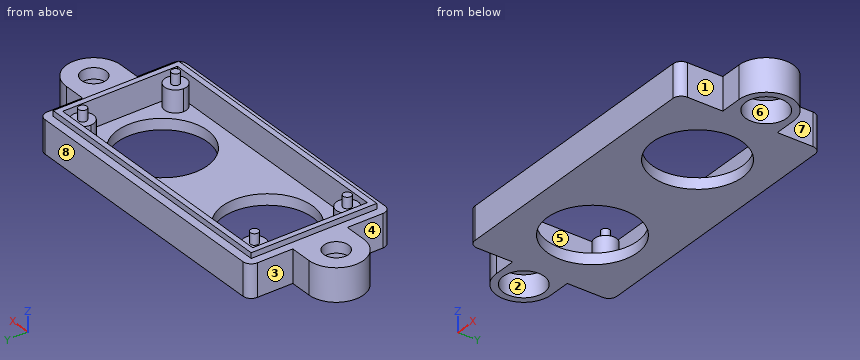
from build123d import *

# Parameters (mm, degrees)
SKETCH011_R             = 2.25
PAD004_DEPTH            = 6
SKETCH021_W             = 49
SKETCH021_H             = 23
SKETCH021_W_2           = 47
SKETCH021_H_2           = 21
PAD005_DEPTH            = 1
SKETCH020_W             = 47
SKETCH020_H             = 21
POCKET005_DEPTH         = 4
SKETCH012_R             = 8.25
POCKET006_DEPTH         = 8
POCKET006_DEPTH_BACK    = 8
SKETCH022_R             = 3.75
POCKET007_DEPTH         = 4
SKETCH024_R             = 2
PAD006_DEPTH            = 6
SKETCH025_R             = 0.75
PAD007_DEPTH            = 2
FILLET001_R             = 1.5
BODY001_PLACEMENT_ANGLE = 180


with BuildPart() as part:
    # Sketch011 → Pad004 (new body)
    with BuildSketch(Plane.XY):
        with BuildLine():
            Line((-26, 13), (26, 13))
            Line((26, 13), (26, 5))
            Line((30, 5), (26, 5))
            ThreePointArc((29.999982, -5), (35, -9e-06), (30, 5))
            Line((29.999982, -5), (25.999982, -5))
            Line((25.999982, -5), (25.999982, -13))
            Line((-26, -13), (25.999982, -13))
            Line((-26, -5), (-26, -13))
            Line((-30, -5), (-26, -5))
            ThreePointArc((-30, 5), (-35, 0), (-30, -5))
            Line((-30, 5), (-26, 5))
            Line((-26, 13), (-26, 5))
        make_face()
        with Locations((-30, 0)):
            Circle(SKETCH011_R, mode=Mode.SUBTRACT)
        with Locations((30, 0)):
            Circle(SKETCH011_R, mode=Mode.SUBTRACT)
    extrude(amount=PAD004_DEPTH)

    # Sketch021 → Pad005 (join, symmetric)
    with BuildSketch(Plane.XY):
        Rectangle(SKETCH021_W, SKETCH021_H)
        Rectangle(SKETCH021_W_2, SKETCH021_H_2, mode=Mode.SUBTRACT)
    extrude(amount=PAD005_DEPTH, both=True)

    # Sketch020 → Pocket005 (cut)
    with BuildSketch(Plane.XY):
        Rectangle(SKETCH020_W, SKETCH020_H)
    extrude(amount=POCKET005_DEPTH, mode=Mode.SUBTRACT)

    # Sketch012 → Pocket006 (cut, two sides)
    with BuildSketch(Plane.XY) as pocket006_sk:
        with Locations((-13, 0)):
            Circle(SKETCH012_R)
        with Locations((13, 0)):
            Circle(SKETCH012_R)
    extrude(amount=-POCKET006_DEPTH, mode=Mode.SUBTRACT)
    extrude(pocket006_sk.sketch, amount=POCKET006_DEPTH_BACK, mode=Mode.SUBTRACT)

    # Sketch022 (on Face5 of Pocket006) → Pocket007 (cut)
    with BuildSketch(Plane.XY.offset(6)):
        with Locations((-30, 0)):
            Circle(SKETCH022_R)
        with Locations((30, 0)):
            Circle(SKETCH022_R)
    extrude(amount=-POCKET007_DEPTH, mode=Mode.SUBTRACT)

    # Sketch024 → Pad006 (join)
    with BuildSketch(Plane.XY):
        with Locations((21.25, 8.5)):
            Circle(SKETCH024_R)
        with Locations((-21.25, 8.5)):
            Circle(SKETCH024_R)
        with Locations((-21.25, -8.5)):
            Circle(SKETCH024_R)
        with Locations((21.25, -8.5)):
            Circle(SKETCH024_R)
    extrude(amount=PAD006_DEPTH)

    # Sketch025 → Pad007 (join)
    with BuildSketch(Plane.XY):
        with Locations((-21.25, 8.5)):
            Circle(SKETCH025_R)
        with Locations((-21.25, -8.5)):
            Circle(SKETCH025_R)
        with Locations((21.25, 8.5)):
            Circle(SKETCH025_R)
        with Locations((21.25, -8.5)):
            Circle(SKETCH025_R)
    extrude(amount=-PAD007_DEPTH)

    # Fillet001
    fillet001_edges = [part.edges().sort_by_distance(p)[0] for p in [
        (26, 13, 3),
        (25.999982, -13, 3),
        (-26, 13, 3),
        (-26, -13, 3),
    ]]
    fillet(fillet001_edges, radius=FILLET001_R)


with BuildPart() as part_1:
    # Body001 placement: moved
    add(part.part.moved(Location((0, 0, -18))).rotate(Axis((0, 0, -18), (0, 1, 0)), BODY001_PLACEMENT_ANGLE))


solid = part_1.part
Here's how the part is built. I have some questions about the finished solid (model axes, mm). Face numbers are marked on the shaded views. A direction names the side the tool comes from. Coordinates: 2 decimals unless noted, no trailing zeros. Write each loop counter-clockwise with the first axis right and the second up, starting at its lowest first coordinate (ties: lowest second). Pieces come first, ordered by that corner, then holes.
Item 1: I want a section at D-D on x = -2. Write out the boundary of the cut face in (y, z), and give its area (3 significant figures).
Item 2: I want a section at C-C on y = 0. Count the separate pieces of the cut face and the enclosed holes in it, and give its area (3 significant figures).
Item 3: Will these pins go through, and if not, where does the flat tip stop? pin 1 (3 mm diameter, centred on x = 28.5, z = -20, fed in from +Y); pin 2 (4.5 mm diameter, centred on x = -27.5, z = -20.5, fed in from +Y); pin 3 (3 mm diameter, centred on y = -10, z = -20.5, fed in from -X).
Item 4: If I drill on line 1 (X direction, y = 0.25, z = -18.5); line 2 (Y direction, x = 6.5, z = -17.5); line 3 (Y direction, x = 30, z = -18.35), over which ranges is the centre line in solid material (lowest first)?
Item 5: I want a section at B-B on z = -22.75. Write out the boundary of the cut face in (x, y).
Item 6: If we mould it in two halves opening along Y, with no side actions, what happens to the marked faces 6, 7 and 8? For each: +Y half, -Y half, draft (parallel to the pull), parting line (faces both ways), or undercut.
Item 7: I want a section at A-A on x = -13. Write out the boundary of the cut face in (y, z), and give its area (3 significant figures).
Item 8: On a 3-axis mill with a long thin cutter (end or side, diameter ignored), from which of +Z, -Z, +X, -X, +Y, -Y can I reach the whole of each face in a straight line? I mean the marked faces 1, 2, 3, 4 and 5. Say none if no direction works.
Findings below:
1. outline: (-13, -24) - (13, -24) - (13, -18) - (11.5, -18) - (11.5, -17) - (10.5, -17) - (10.5, -22) - (-10.5, -22) - (-10.5, -17) - (-11.5, -17) - (-11.5, -18) - (-13, -18) - close
1. area: 74.0 mm2
2. separate pieces: 5
2. enclosed holes: 0
2. area: 90.0 mm2
3. pin 1: stops at y = 5
3. pin 2: stops at y = 12.8
3. pin 3: stops at x = -26
4. line 1: x = -34.99 to -32.24, -27.76 to -23.5, 23.5 to 27.76, 32.24 to 34.99
4. line 2: y = -11.5 to -10.5, 10.5 to 11.5
4. line 3: y = -5 to -2.25, 2.25 to 5
5. outline: (-30, -5) - (-26, -5) - (-26, -11.5) arc R1.5 ccw to (-24.5, -13) - (24.5, -13) arc R1.5 ccw to (26, -11.5) - (26, -5) - (30, -5) arc R5 ccw to (30, 5) - (26, 5) - (26, 11.5) arc R1.5 ccw to (24.5, 13) - (-24.5, 13) arc R1.5 ccw to (-26, 11.5) - (-26, 5) - (-30, 5) arc R5 ccw to start; hole circle Ø7.5 at (-30, 0); hole circle Ø16.5 at (-13, 0); hole circle Ø16.5 at (13, 0); hole circle Ø7.5 at (30, 0)
6. face 6: undercut
6. face 7: draft
6. face 8: +Y half
7. outline: (-13, -24) - (-8.25, -24) - (-8.25, -22) - (-10.5, -22) - (-10.5, -17) - (-11.5, -17) - (-11.5, -18) - (-13, -18) - close; (8.25, -24) - (13, -24) - (13, -18) - (11.5, -18) - (11.5, -17) - (10.5, -17) - (10.5, -22) - (8.25, -22) - close
7. area: 41.0 mm2
8. face 1: +Z, -Z, +X, -Y
8. face 2: -Z
8. face 3: +Z, -Z, -X, +Y
8. face 4: +Z, -Z, -X, -Y
8. face 5: +Z
